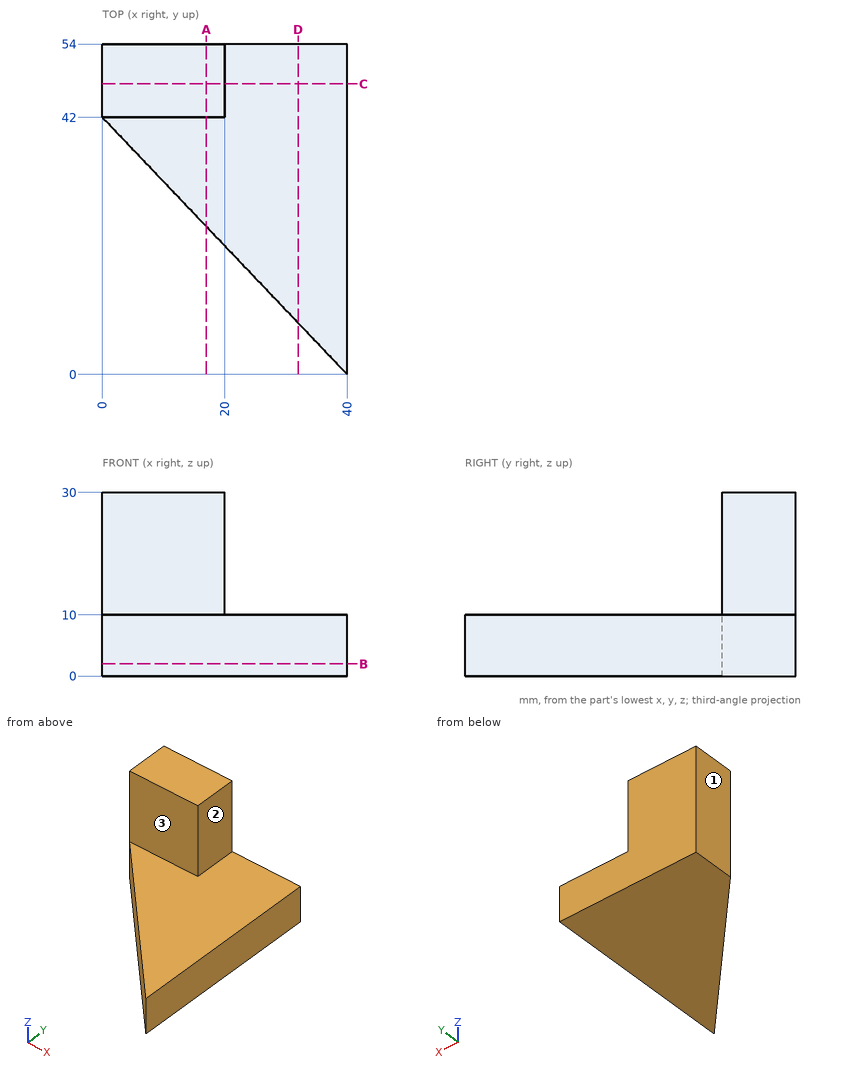
The figure shows three views and two pictorial views of one solid part (mm, origin at its lowest corner). Answer the questions. A direction names the side the tool comes from. Round coordinates to 2 decimals unless told otherwise and drop trailing zeros. Loops run counter-clockwise (first coordinate to the right, second up) from the corner with the lowest first, then second, coordinate; pieces in that order, holes last. Notation, with made-up numbers: (37.25, 14.25) - (73.25, 14.25) arc R27 cw to (73.25, 47.25) - close; hole circle Ø7 at (55, 82.5). An arc over 180 degrees is marked (long way). Use one line per item in the form item = value. Start each with the question number.
(1) Find section D-D on x = 32. Determine the outline of the cut face in (y, z), and give its area (3 significant figures).
(2) Flat-ended cylindrical pins translate along their axes: P1, Ø1, axis at y = 47.5, z = 12.5, coming from the +X side; P2, Ø12, axis at x = 14, z = 7, coming from the -Y side; P3, Ø6, axis at x = 8, z = 16.5, coming from the -Y side. Find the tip coordinate at first contact, or state that the pin passes through.
(3) Consider line 1 (Y direction, x = 5.5, z = 21.25); line 2 (Z direction, x = 36, y = 33); line 3 (X direction, y = 42.5, z = 14). Determine where each line is inside the solid, lowest interval first.
(4) Find section C-C on y = 47.5. Determine the outline of the cut face in (x, z), and give its area (3 significant figures).
(5) Find section A-A on x = 17. Determine the outline of the cut face in (y, z), and give its area (4 significant figures).
(6) Find section B-B on z = 2. Determine the outline of the cut face in (x, y).
(7) Which of the six approach directions +Z, -Z, +X, -X, +Y, -Y give full straight-line access (tool end or side, diameter ignored) to the marked faces 1, 2 and 3?
Answer list:
q1.outline = (8.4, 0) - (54, 0) - (54, 10) - (8.4, 10) - close
q1.area = 456 mm^2
q2.P1 = 20
q2.P2 = 21
q2.P3 = 42
q3.line_1 = 42 to 54
q3.line_2 = 0 to 10
q3.line_3 = 0 to 20
q4.outline = (0, 0) - (40, 0) - (40, 10) - (20, 10) - (20, 30) - (0, 30) - close
q4.area = 800 mm^2
q5.outline = (24.15, 0) - (54, 0) - (54, 30) - (42, 30) - (42, 10) - (24.15, 10) - close
q5.area = 538.5 mm^2
q6.outline = (0, 42) - (40, 0) - (40, 54) - (0, 54) - close
q7.face_1 = +Z, -Z, -X, +Y, -Y
q7.face_2 = +Z, +X, +Y, -Y
q7.face_3 = +Z, +X, -X, -Y
